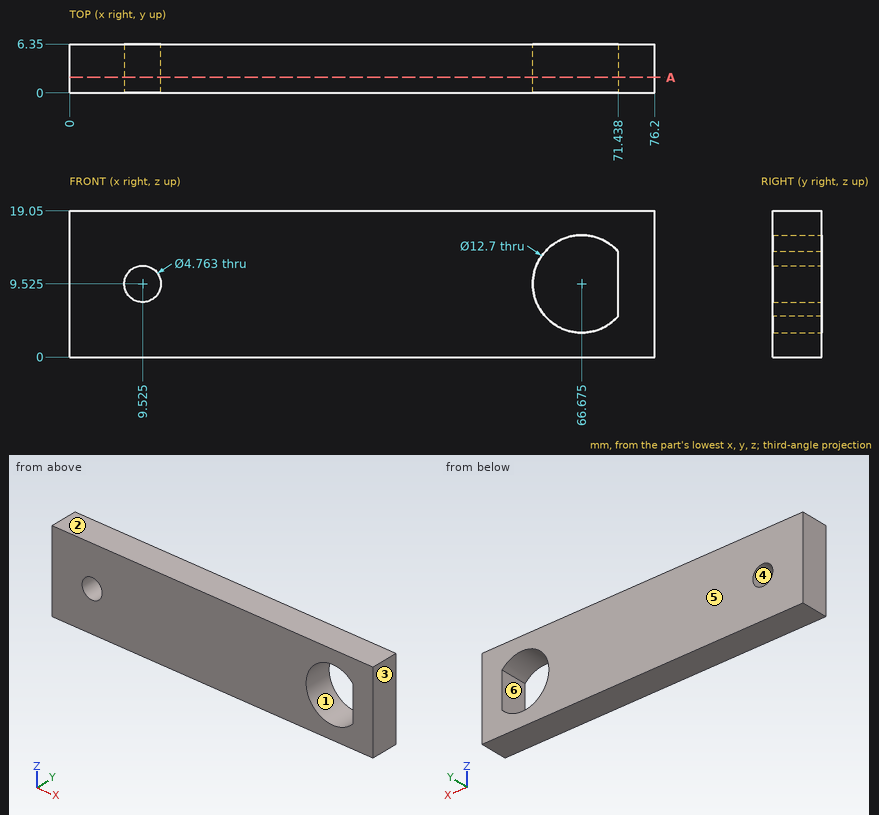
Verification items for this drawing (mm, ordinates from the low corner). A direction names the side the tool comes from. Coordinates: 2 decimals unless noted, no trailing zeros.
Item 1: Sectioned sample at A-A, the plane y = 2. Count the separate pieces of the cut face and the enclosed holes in it, then the cut area to 3 significant figures.
Item 2: Thickness scan on line 1 (X direction, y = 2.5, z = 8.25) (1 decimal); line 2 (X direction, y = 3.5, z = 7.5) (1 decimal); line 3 (X direction, y = 1.75, z = 14). Record the ranges inside material, lowest first.
Item 3: Release check for a two-part mould opening along X. For the marked faces 1, 2, 3 and 4 record: released by +X, released by -X, zero draft, split by the parting line, or undercut.
Item 4: Access from +Z, -Z, +X, -X, +Y, -Y to the whole of each face (thin tool, end or side, straight path). Record for the marked faces 5 and 6.
Check result:
1. separate pieces: 1
1. enclosed holes: 2
1. area: 1,320 mm2
2. line 1: x = 0 to 7.5, 11.5 to 60.5, 71.4 to 76.2
2. line 2: x = 0 to 8.3, 10.8 to 60.7, 71.4 to 76.2
2. line 3: x = 0 to 62.17, 71.18 to 76.2
3. face 1: undercut
3. face 2: zero draft
3. face 3: released by +X
3. face 4: undercut
4. face 5: +Z, -Z, +X, -X, +Y
4. face 6: +Y, -Y
